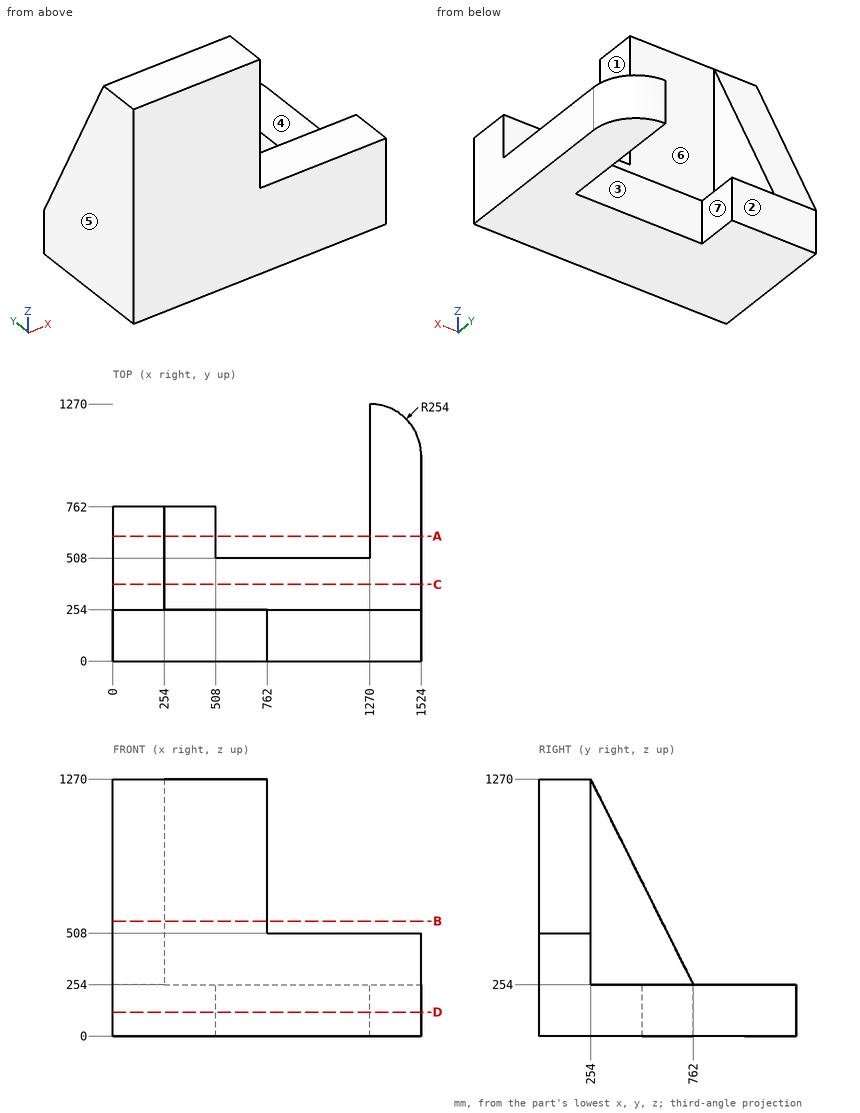
Drawing for the job (mm, zero at the part's lowest x, y, z). A direction names the side the tool comes from. Coordinates: 2 decimals unless noted, no trailing zeros. Order: outer loops, then holes, each group sorted by start corner. A loop starts at its lowest first (then second) coordinate and runs counter-clockwise, first axis right, second up.
Item 1: Band-saw the part on A-A on y = 617.5. List the corners of the cut face in (x, z), plus the area to 3 significant figures.
Check sheet entries:
outline: (0, 0) - (508, 0) - (508, 254) - (254, 254) - (254, 543) - (0, 543) - close; (1270, 0) - (1524, 0) - (1524, 254) - (1270, 254) - close
area: 267,000 mm2
Item 2: Band-saw the part on D-D on z = 117.5. List the corners of the cut face in (x, y), plus the area to 3 significant figures.
Check sheet entries:
outline: (0, 0) - (1524, 0) - (1524, 1016) arc R254 ccw to (1270, 1270) - (1270, 508) - (508, 508) - (508, 762) - (0, 762) - close
area: 1,080,000 mm2
Item 3: Band-saw the part on C-C on y = 379. List the corners of the cut face in (x, z).
Check sheet entries:
outline: (0, 0) - (1524, 0) - (1524, 254) - (254, 254) - (254, 1020) - (0, 1020) - close
Item 4: 3-axis set-ups, long thin cutter, end or side, ignore diameter. For the marked faces 1, 2, 3 and 4: which of +Z, -Z, +X, -X, +Y, -Y reach the whole face in a straight line?
Check sheet entries:
face 1: +Z, +X, +Y, -Y
face 2: +Z, -Z, -X, +Y
face 3: +Z, -Z, +Y
face 4: +Z, +X, +Y
Item 5: Pin check, flat tip, straight feed: pin 1 Ø4 at (x, z) = (686.5, 557.5) entering from +Y. Stop position of the tip, or through.
Check sheet entries:
pin 1: stops at y = 254
Item 6: Drill centre lines: L1, parallel to Y at x = 671, z = 881; L2, parallel to X at y = 192.5, z = 712. Where is each one in solid material? Low to high.
Check sheet entries:
L1: y = 0 to 254
L2: x = 0 to 762
Item 7: Two-plate mould, pull along X, no slides. Class the marked faces 5, 6 and 7: +X half, -X half, draft (parallel to the pull), parting line (faces both ways), or undercut.
Check sheet entries:
face 5: -X half
face 6: draft
face 7: undercut
Item 8: Band-saw the part on B-B on z = 567.5. List the corners of the cut face in (x, y), plus the area to 3 significant figures.
Check sheet entries:
outline: (0, 0) - (762, 0) - (762, 254) - (254, 254) - (254, 605.25) - (0, 605.25) - close
area: 283,000 mm2
